```python
from build123d import *

# Parameters (mm, degrees)
SKETCH_1_R          = 15
EXTRUDE_1_DEPTH     = 5
EXTRUDE_2_DEPTH     = 5
SKETCH_3_R          = 2
CUT_EXTRUDE_1_DEPTH = 5


with BuildPart() as part:
    # 草图1 → 凸台-拉伸1 (new body)
    with BuildSketch(Plane.XY):
        Circle(SKETCH_1_R)
    extrude(amount=EXTRUDE_1_DEPTH)

    # 草图2 → 凸台-拉伸2 (add)
    with BuildSketch(Plane(origin=(0, 0, 0), x_dir=(-1, 0, 0), z_dir=(0, 0, -1))):
        with BuildLine():
            Line((-2.565151075, 7.047694656), (-4.275251792, 11.74615776))
            ThreePointArc((-4.275251792, 11.74615776), (0, 12.5), (4.275251792, 11.74615776))
            Line((4.275251792, 11.74615776), (2.565151075, 7.047694656))
            ThreePointArc((2.565151075, 7.047694656), (0, 7.5), (-2.565151075, 7.047694656))
        make_face()
        with BuildLine():
            Line((7.047694656, 2.565151075), (11.74615776, 4.275251792))
            ThreePointArc((11.74615776, 4.275251792), (12.5, 0), (11.74615776, -4.275251792))
            Line((11.74615776, -4.275251792), (7.047694656, -2.565151075))
            ThreePointArc((7.047694656, -2.565151075), (7.5, 0), (7.047694656, 2.565151075))
        make_face()
        with BuildLine():
            Line((2.565151075, -7.047694656), (4.275251792, -11.74615776))
            ThreePointArc((4.275251792, -11.74615776), (0, -12.5), (-4.275251792, -11.74615776))
            Line((-4.275251792, -11.74615776), (-2.565151075, -7.047694656))
            ThreePointArc((-2.565151075, -7.047694656), (0, -7.5), (2.565151075, -7.047694656))
        make_face()
        with BuildLine():
            Line((-7.047694656, -2.565151075), (-11.74615776, -4.275251792))
            ThreePointArc((-11.74615776, -4.275251792), (-12.5, 0), (-11.74615776, 4.275251792))
            Line((-11.74615776, 4.275251792), (-7.047694656, 2.565151075))
            ThreePointArc((-7.047694656, 2.565151075), (-7.5, 0), (-7.047694656, -2.565151075))
        make_face()
    extrude(amount=EXTRUDE_2_DEPTH)

    # 草图3 → 切除-拉伸1 (cut)
    with BuildSketch(Plane(origin=(0, 0, 0), x_dir=(-1, 0, 0), z_dir=(0, 0, -1))):
        Circle(SKETCH_3_R)
    extrude(amount=-CUT_EXTRUDE_1_DEPTH, mode=Mode.SUBTRACT)


solid = part.part
```
Verification items for the finished model (mm, model axes). A direction names the side the tool comes from. Give positions to 0.01 mm unless a question says otherwise; leave off trailing zeros. Write each loop counter-clockwise with the first axis right and the second up, starting at its lowest first coordinate (ties: lowest second). Pieces come first, ordered by that corner, then holes. Notation, with made-up numbers: (13, 7.5) - (23, 7.5) arc R20 cw to (23, 24.5) - close; hole circle Ø11 at (-31, 48). An arc over 180 degrees is marked (long way). Put each result on its own line as item: value.
Q1. Set-up check for faces 1 (the face through (0, 7.5, -2.5)), 2 (the face through (-0.1, -12.5, -2.5)), 3 (the face through (3.408, 9.364, -2.465)), 4 (the face through (0.1, 12.5, -2.5)): record each of +Z, -Z, +X, -X, +Y, -Y from which the full face is reachable in a straight line by a thin tool's end or side.
Result:
face 1: -Z
face 2: -Z, -Y
face 3: -Z, +X
face 4: -Z, +Y
Q2. Section check B-B on y = 0. Record the cut outline in (x, z), and give its area (3 significant figures).
Result:
outline: (-15, 0) - (-12.5, 0) - (-12.5, -5) - (-7.5, -5) - (-7.5, 0) - (-2, 0) - (-2, 5) - (-15, 5) - close; (2, 0) - (7.5, 0) - (7.5, -5) - (12.5, -5) - (12.5, 0) - (15, 0) - (15, 5) - (2, 5) - close
area: 180 mm2
Q3. Mould release check, pull along Y, two halves, no side actions. Record for faces 5 (the face through (-3.408, -9.364, -2.465)), 6 (the face through (-9.43, -3.432, -2.465)), 7 (the face through (3, 0, 5)): released by +Y, released by -Y, zero draft, split by the parting line, or undercut.
Result:
face 5: undercut
face 6: released by -Y
face 7: zero draft
Q4. Scan lines: probe 1 along Y at (x, z) = (0, 3.2); probe 2 along Z at (x, y) = (-10, -6.75); probe 3 along Y at (x, z) = (1.25, 4). Record each from-to range of solid material in increasing order. Write a range as from..to.
Result:
probe 1: -15..-2, 2..15
probe 2: 0..5
probe 3: -14.95..-1.56, 1.56..14.95
Q5. Section check D-D on x = 3. Record the cut outline in (y, z).
Result:
outline: (-14.7, 0) - (-12.13, 0) - (-12.13, -5) - (-8.24, -5) - (-8.24, 0) - (8.24, 0) - (8.24, -5) - (12.13, -5) - (12.13, 0) - (14.7, 0) - (14.7, 5) - (-14.7, 5) - close
Q6. Section check A-A on z = -2.75. Record the cut outline in (x, y).
Result:
outline: (-11.75, -4.28) - (-7.05, -2.57) arc R7.5 cw to (-7.05, 2.57) - (-11.75, 4.28) arc R12.5 ccw to start; (-4.28, -11.75) arc R12.5 ccw to (4.28, -11.75) - (2.57, -7.05) arc R7.5 cw to (-2.57, -7.05) - close; (-4.28, 11.75) - (-2.57, 7.05) arc R7.5 cw to (2.57, 7.05) - (4.28, 11.75) arc R12.5 ccw to start; (7.05, -2.57) - (11.75, -4.28) arc R12.5 ccw to (11.75, 4.28) - (7.05, 2.57) arc R7.5 cw to start
Q7. Depth check by flat-ended pin: P1, Ø2, axis at y = 7.5, z = -0.5, coming from the +X side; P2, Ø3, axis at y = 7.5, z = 1.5, coming from the -X side; P3, Ø3, axis at x = -1, y = -1, coming from the -Z side. Enter the tip coordinate at first touch or a pass-through.
Result:
P1: x = 13.45
P2: x = -13.75
P3: z = 0
